```python
from build123d import *

# Parameters (mm, degrees)
SKETCH1_W           = 70
SKETCH1_H           = 70
BOSS_EXTRUDE1_DEPTH = 5
SKETCH7_R           = 0.75
CUT_EXTRUDE1_DEPTH  = 6


with BuildPart() as part:
    # Sketch1 → Boss-Extrude1 (new body)
    with BuildSketch(Plane(origin=(0, 0, 0), x_dir=(1, 0, 0), z_dir=(0, 1, 0))):
        Rectangle(SKETCH1_W, SKETCH1_H)
    extrude(amount=-BOSS_EXTRUDE1_DEPTH)

    # Sketch7 → Cut-Extrude1 (cut, through all)
    with BuildSketch(Plane(origin=(0, 0, 0), x_dir=(1, 0, 0), z_dir=(0, 1, 0))):
        with Locations((0, 15)):
            Circle(SKETCH7_R)
        with Locations((0, -15)):
            Circle(SKETCH7_R)
    extrude(amount=-CUT_EXTRUDE1_DEPTH, mode=Mode.SUBTRACT)


solid = part.part
```
Can you work these out from the model? Positions are in its coordinate system, mm. Coordinates: 2 decimals unless noted, no trailing zeros. Write item = value, one per line. Start each with the question number.
Q1. I'm going to push a flat-ended pin straight in: pin 1 (0.9 mm diameter, centred on x = 0, z = -15, fed in from -Y) (3 decimals). Where does the tip first touch, or does it pass through?
Q2. Thinking about a two-plate mould opening in X: for faces 1 (the face through (0, 0, 0)), 2 (the face through (-35, -2, 0)), 3 (the face through (-0.098, -2.465, -15.744)), which applies, released by +X, released by -X, zero draft, split by the parting line, or undercut?
Q3. If I drill on L1, parallel to Z at x = 0, y = -3.1; L2, parallel to X at y = -2.05, z = -15, over which ranges is the centre line in solid material (lowest first)? Write a range as [from, to].
Check sheet entries:
q1.pin_1 = through
q2.face_1 = zero draft
q2.face_2 = released by -X
q2.face_3 = undercut
q3.L1 = [-35, -15.75], [-14.25, 14.25], [15.75, 35]
q3.L2 = [-35, -0.75], [0.75, 35]
